CAD build for the part. Positions are in the model's coordinates, mm. Face numbers are marked on the shaded views. A direction names the side the tool comes from. Coordinates: 2 decimals unless noted, no trailing zeros. Write each loop counter-clockwise with the first axis right and the second up, starting at its lowest first coordinate (ties: lowest second). Pieces come first, ordered by that corner, then holes.
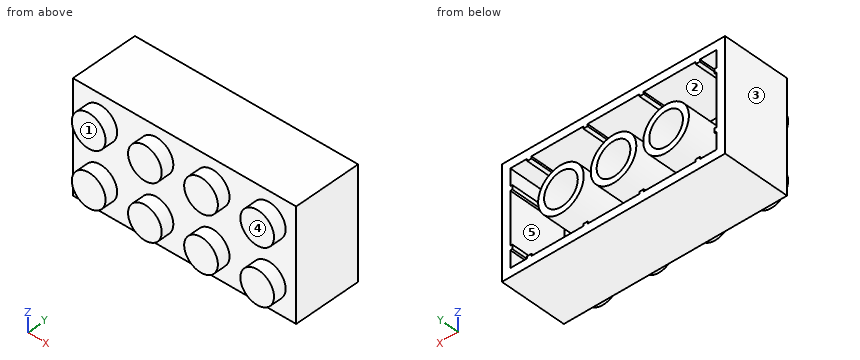
```python
from build123d import *

# Parameters (mm, degrees)
F0_W     = 31.8
F0_H     = 15.8
F1_DEPTH = 9.6
F2_R     = 2.4
F3_DEPTH = 1.8
F5_T     = -1.2
F4_R     = 3.25
F4_R_2   = 2.4
F6_DEPTH = 9.6
F7_W     = 0.6
F7_H     = 0.3
F7_W_2   = 0.3
F7_H_2   = 0.6
F8_DEPTH = 9.6


with BuildPart() as f1:
    # F0 (on Front) → F1 (new body)
    with BuildSketch(Plane.XZ):
        Rectangle(F0_W, F0_H)
    extrude(amount=F1_DEPTH)

    # F2 (on face) → F3 (join)
    with BuildSketch(Plane.XZ.offset(9.6)):
        with Locations((-12, 4)):
            Circle(F2_R)
        with Locations((-4, 4)):
            Circle(F2_R)
        with Locations((4, 4)):
            Circle(F2_R)
        with Locations((12, 4)):
            Circle(F2_R)
        with Locations((-12, -4)):
            Circle(F2_R)
        with Locations((-4, -4)):
            Circle(F2_R)
        with Locations((4, -4)):
            Circle(F2_R)
        with Locations((12, -4)):
            Circle(F2_R)
    extrude(amount=F3_DEPTH)

    # F5
    f5_openings = [f1.faces().sort_by_distance(p)[0] for p in [
        (0, 0, 0),
    ]]
    offset(amount=F5_T, openings=f5_openings, kind=Kind.INTERSECTION)

    # F4 (on face) → F6 (join)
    with BuildSketch(Plane(origin=(0, 0, 0), x_dir=(-1, 0, 0), z_dir=(0, 1, 0))):
        with Locations((7.49, 0)):
            Circle(F4_R)
        with Locations((7.49, 0)):
            Circle(F4_R_2, mode=Mode.SUBTRACT)
        Circle(F4_R)
        Circle(F4_R_2, mode=Mode.SUBTRACT)
        with Locations((-7.49, 0)):
            Circle(F4_R)
        with Locations((-7.49, 0)):
            Circle(F4_R_2, mode=Mode.SUBTRACT)
    extrude(amount=-F6_DEPTH)

    # F7 (on face) → F8 (join)
    with BuildSketch(Plane(origin=(0, 0, 0), x_dir=(-1, 0, 0), z_dir=(0, 1, 0))):
        with Locations((4, -6.55)):
            Rectangle(F7_W, F7_H)
        with Locations((-4, -6.55)):
            Rectangle(F7_W, F7_H)
        with Locations((-12, -6.55)):
            Rectangle(F7_W, F7_H)
        with Locations((-14.55, -4)):
            Rectangle(F7_W_2, F7_H_2)
        with Locations((-14.55, 4)):
            Rectangle(F7_W_2, F7_H_2)
        with Locations((-12, 6.55)):
            Rectangle(F7_W, F7_H)
        with Locations((-4, 6.55)):
            Rectangle(F7_W, F7_H)
        with Locations((4, 6.55)):
            Rectangle(F7_W, F7_H)
        with Locations((12, 6.55)):
            Rectangle(F7_W, F7_H)
        with Locations((12, -6.55)):
            Rectangle(F7_W, F7_H)
        with Locations((14.55, -4)):
            Rectangle(F7_W_2, F7_H_2)
        with Locations((14.55, 4)):
            Rectangle(F7_W_2, F7_H_2)
    extrude(amount=-F8_DEPTH)


solid = f1.part
```
Item 1: Saw through at C-C, the plane z = -5.5. Write the cut outline in (x, y).
Item 2: Two-plate mould, pull along X, no slides. Class the marked faces 1, 2 and 3: +X half, -X half, draft (parallel to the pull), parting line (faces both ways), or undercut.
Item 3: Flat gauge pins, fed straight in: pin 1 Ø4.5 at (x, z) = (7.49, 0) entering from +Y; pin 2 Ø1.4 at (x, z) = (4, 4) entering from +Y. Where does each tip first touch, or does it go through?
Item 4: Wall check: line 1 along X through (y, z) = (-9.35, -4); line 2 along Z through (x, y) = (-4, -9.25); line 3 along X through (y, z) = (-8, 6.25). Give the ranges that are in metal, low to high.
Item 5: Saw through at B-B, the plane y = -0.75. State how many separate pieces and enclosed holes the cut face has, and give its area (3 significant figures).
Item 6: Which spindle directions (+Z, -Z, +X, -X, +Y, -Y) get a long thin tool onto all of the face, cutting with end or side? Do the marked faces 4 and 5. Say none if no direction does.
Item 7: Saw through at A-A, the plane x = 12. Write the cut outline in (y, z), and give its area (3 significant figures).
Item 8: Saw through at D-D, the plane x = 0. Write the cut outline in (y, z), and give its area (3 significant figures).
Working result:
1. outline: (-15.9, -9.6) - (-13.87, -9.6) - (-13.87, -11.4) - (-10.13, -11.4) - (-10.13, -9.6) - (-5.87, -9.6) - (-5.87, -11.4) - (-2.13, -11.4) - (-2.13, -9.6) - (2.13, -9.6) - (2.13, -11.4) - (5.87, -11.4) - (5.87, -9.6) - (10.13, -9.6) - (10.13, -11.4) - (13.87, -11.4) - (13.87, -9.6) - (15.9, -9.6) - (15.9, 0) - (14.7, 0) - (14.7, -8.4) - (-14.7, -8.4) - (-14.7, 0) - (-15.9, 0) - close
2. face 1: draft
2. face 2: undercut
2. face 3: -X half
3. pin 1: stops at y = -8.4
3. pin 2: stops at y = -10.2
4. line 1: x = -15.9 to -13.2, -10.8 to -5.2, -2.8 to 2.8, 5.2 to 10.8, 13.2 to 15.9
4. line 2: z = -7.9 to -5.2, -2.8 to 2.8, 5.2 to 7.9
4. line 3: x = -15.9 to -14.7, 14.7 to 15.9
5. separate pieces: 4
5. enclosed holes: 4
5. area: 156 mm2
6. face 4: +Z, -Z, +X, -X, -Y
6. face 5: +Y
7. outline: (-11.4, -6.4) - (-9.6, -6.4) - (-9.6, -7.9) - (0, -7.9) - (0, -6.4) - (-8.4, -6.4) - (-8.4, -5.2) - (-10.2, -5.2) - (-10.2, -2.8) - (-8.4, -2.8) - (-8.4, 2.8) - (-10.2, 2.8) - (-10.2, 5.2) - (-8.4, 5.2) - (-8.4, 6.4) - (0, 6.4) - (0, 7.9) - (-9.6, 7.9) - (-9.6, 6.4) - (-11.4, 6.4) - (-11.4, 1.6) - (-9.6, 1.6) - (-9.6, -1.6) - (-11.4, -1.6) - close
7. area: 52.8 mm2
8. outline: (-9.6, -7.9) - (0, -7.9) - (0, -6.7) - (-8.4, -6.7) - (-8.4, -3.25) - (0, -3.25) - (0, -2.4) - (-8.4, -2.4) - (-8.4, 2.4) - (0, 2.4) - (0, 3.25) - (-8.4, 3.25) - (-8.4, 6.7) - (0, 6.7) - (0, 7.9) - (-9.6, 7.9) - close
8. area: 53.4 mm2
